```python
from build123d import *

# Parameters (mm, degrees)
F0_W            = 165.4
F0_H            = 15
F0_W_2          = 9.8
F1_DEPTH        = 6
F2_DEPTH        = 4
F4_D            = 2.5
F4_DEPTH        = 200
F5_R            = 2
F7_W            = 6.5
F7_H            = 6
F8_DEPTH        = 2
F9_W            = 172
F9_H            = 2
F10_DEPTH       = 5
F11_SIZE2       = 3
F11_SIZE        = 1.5
F13_D           = 3
F13_DEPTH       = 4
F13_CSINK_D     = 7
F13_CSINK_ANGLE = 90


with BuildPart() as f1:
    # F0 (on Top) → F1 (new body)
    with BuildSketch(Plane.XY):
        with Locations((-2.652436, -0.515384)):
            Rectangle(F0_W, F0_H)
        with Locations((-90.252436, -0.515384)):
            Rectangle(F0_W_2, F0_H)
        with Locations((84.947564, -0.515384)):
            Rectangle(F0_W_2, F0_H)
    extrude(amount=F1_DEPTH)

    # F0 (on Top) → F2 (cut)
    with BuildSketch(Plane.XY):
        with Locations((-2.652436, -0.515384)):
            Rectangle(F0_W, F0_H)
    extrude(amount=F2_DEPTH, mode=Mode.SUBTRACT)

    # F4
    with Locations(Plane(origin=(-95.152436, 0, 0), x_dir=(0, -1, 0), z_dir=(-1, 0, 0))):
        with Locations((2.015384, 3)):
            Hole(F4_D / 2, depth=F4_DEPTH)

    # F5
    f5_edges = [f1.edges().sort_by_distance(p)[0] for p in [
        (84.947564, 6.984616, 0),
        (-90.252436, 6.984616, 0),
        (-90.252436, -8.015384, 0),
        (84.947564, -8.015384, 0),
    ]]
    fillet(f5_edges, radius=F5_R)

    # F7 (on face) → F8 (cut)
    with BuildSketch(Plane.XY.offset(6)):
        with Locations((-91.902436, 3.984616)):
            Rectangle(F7_W, F7_H)
        with Locations((86.597564, 3.984616)):
            Rectangle(F7_W, F7_H)
    extrude(amount=-F8_DEPTH, mode=Mode.SUBTRACT)

    # F9 (on face) → F10 (join)
    with BuildSketch(Plane(origin=(0, 6.984616, 0), x_dir=(-1, 0, 0), z_dir=(0, 1, 0))):
        with Locations((2.652436, 5)):
            Rectangle(F9_W, F9_H)
    extrude(amount=F10_DEPTH)

    # F11
    f11_edges = [f1.edges().sort_by_distance(p)[0] for p in [
        (-2.652436, 11.984616, 4),
    ]]
    chamfer(f11_edges, length=F11_SIZE, length2=F11_SIZE2)

    # F13
    with Locations(Plane.XY.offset(6)):
        with Locations((-79.352436, -2.015384), (-38.352436, -2.015384), (-2.652436, -2.015384), (33.047564, -2.015384), (74.047564, -2.015384)):
            CounterSinkHole(F13_D / 2, F13_CSINK_D / 2, depth=F13_DEPTH, counter_sink_angle=F13_CSINK_ANGLE)


solid = f1.part
```
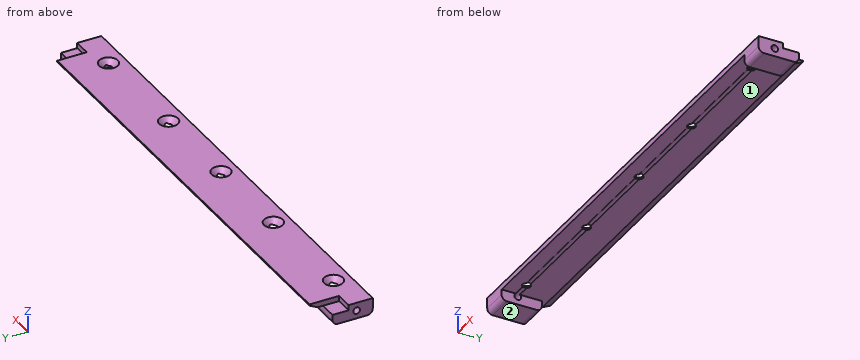
Can you work these out from the model? Positions are in its coordinate system, mm. Face numbers are marked on the shaded views. Give positions to 0.01 mm unless a question says otherwise; leave off trailing zeros. Order: outer loops, then holes, each group sorted by start corner. A loop starts at its lowest first (then second) coordinate and runs counter-clockwise, first axis right, second up. Notation, with made-up numbers: M -38,-26.75 L -30,-26.75 A4 ccw -30,-19.75 Z; hole C 89,47 d4. An arc over 180 degrees is marked long. One line per item, written item: value.
1) For P1, Ø5, axis at x = -92.5, y = 5, coming from the +Z side; P2, Ø1.6, axis at x = -14, y = -4, coming from the -Z side; P3, Ø2, axis at x = -88, z = 3.5, coming from the +Y side, each with a flat end and sliding along its axis, tell me the tip position at first contact or that it passes through.
Answer sheet:
P1: stops at z = 4
P2: stops at z = 4
P3: stops at y = 9.98
2) I want a section at B-B, the plane x = -52. List the corners of the cut face in (y, z) for me.
Answer sheet:
outline: M -8.02,4 L -2.77,4 A1.25 cw -1.27,4 L 8.98,4 L 11.98,5.5 L 11.98,6 L -8.02,6 Z
3) I want a section at A-A, the plane z = 3. List the corners of the cut face in (x, y) for me.
Answer sheet:
outline: M -95.15,-8.02 L -85.35,-8.02 L -85.35,-3.27 L -95.15,-3.27 Z; M -95.15,-0.77 L -85.35,-0.77 L -85.35,6.98 L -95.15,6.98 Z; M 80.05,-8.02 L 89.85,-8.02 L 89.85,-3.27 L 80.05,-3.27 Z; M 80.05,-0.77 L 89.85,-0.77 L 89.85,6.98 L 80.05,6.98 Z
4) Please list where these lines run through material, in increasing order: line 1 along X through (y, z) = (0, 1.5); line 2 along Y through (x, z) = (-86, 3); line 3 along Z through (x, y) = (-23.5, 8).
Answer sheet:
line 1: x = -95.15 to -85.35, 80.05 to 89.85
line 2: y = -8.02 to -3.27, -0.77 to 6.98
line 3: z = 4 to 6
5) We'd pull the mould along X, two halves only. Please class the marked faces 1 and 2: released by +X, released by -X, zero draft, split by the parting line, or undercut.
Answer sheet:
face 1: undercut
face 2: zero draft
